For this review, take the finished solid that the model builds, in its own axes (mm). A direction names the side the tool comes from. Give positions to 0.01 mm unless a question says otherwise; leave off trailing zeros. Write each loop counter-clockwise with the first axis right and the second up, starting at its lowest first coordinate (ties: lowest second). Pieces come first, ordered by that corner, then holes.
Q1. Mouldability with a two-part tool opening along X and no side actions: class faces 3 (the cylindrical face through (-2.909, 0.042, -2.202)), 4 (the cylindrical face through (-5.58, 0.04, 0.02)), 5 (the flat face through (0, -3, 0)) as released by +X, released by -X, zero draft, split by the parting line, or undercut.
Q2. Insertion check: P1, Ø3, axis at x = -1, z = 0, coming from the -Y side; P2, Ø2, axis at x = -4.5, z = -2.5, coming from the -Y side; P3, Ø2, axis at x = -0.5, y = 9.5, coming from the -Z side; P4, Ø1, axis at x = -2.5, y = 0, coming from the +Z side. Each pin has a flat end and moves straight along its axis. Give the tip position at first contact, or say it passes through.
Q3. We need section C-C (y = 3.5). Write out the cut boundary in (x, z) (3 decimals).
Q4. Machinability: for faces 1 (the flat face through (-5, -3, 0)), 2 (the flat face through (-2, 3, 0)), which of the approach directions +Z, -Z, +X, -X, +Y, -Y give a long, thin tool a straight path to every point of the face, cutting with its end or side? Answer none if there is none.
Q5. For line 1 (Y direction, x = -1.5, z = -3.75); line 2 (Z direction, x = -6, y = 9); line 3 (Z direction, x = -1.25, y = 9.25), list the stretches that pass through material, from the lowest coordinate up.
Q6. We need section B-B (y = -1.5). Write out the cut boundary in (x, z).
Q7. We need section A-A (x = -2.54). Write out the cut boundary in (y, z) (3 decimals).
Q8. We need section D-D (z = -2.54). Write out the cut boundary in (x, y).
```python
from build123d import *

# Parameters (mm, degrees)
BOSS_EXTRUDE_1_DEPTH = 8.7
SKETCH_2_R           = 0.5
BOSS_EXTRUDE_2_DEPTH = 6


with BuildPart() as part:
    # Sketch 1 → Boss-Extrude 1 (new body)
    with BuildSketch(Plane.ZX.offset(3)):
        with BuildLine():
            Line((-0.13, 1.4), (2.03, 1.4))
            Line((2.03, 1.4), (2.03, -6.47))
            Line((2.03, -6.47), (-0.13, -6.47))
            ThreePointArc((-0.13, -6.47), (-4.065, -2.535), (-0.13, 1.4))
        make_face()
    extrude(amount=BOSS_EXTRUDE_1_DEPTH)

    # Sketch 2 → Boss-Extrude 2 (add)
    with BuildSketch(Plane.XZ.offset(-3)):
        Circle(SKETCH_2_R)
        with Locations((-2.54, -2.54)):
            Circle(SKETCH_2_R)
        with Locations((-5.08, 0)):
            Circle(SKETCH_2_R)
    extrude(amount=BOSS_EXTRUDE_2_DEPTH)


solid = part.part
```
Computed:
1. face 3: split by the parting line
1. face 4: undercut
1. face 5: zero draft
2. P1: stops at y = -3
2. P2: stops at y = 3
2. P3: stops at z = -3.93
2. P4: stops at z = -2.04
3. outline: (-6.47, -0.13) arc R3.935 ccw to (1.4, -0.13) - (1.4, 2.03) - (-6.47, 2.03) - close
4. face 1: +Z, -Z, +X, -X, -Y
4. face 2: -Y
5. line 1: y = 3 to 11.7
5. line 2: z = -1.99 to 2.03
5. line 3: z = -3.85 to 2.03
6. outline: circle Ø1 at (-5.08, 0); circle Ø1 at (-2.54, -2.54); circle Ø1 at (0, 0)
7. outline: (-3, -3.04) - (3, -3.04) - (3, -4.065) - (11.7, -4.065) - (11.7, 2.03) - (3, 2.03) - (3, -2.04) - (-3, -2.04) - close
8. outline: (-5.65, 3) - (-3.04, 3) - (-3.04, -3) - (-2.04, -3) - (-2.04, 3) - (0.58, 3) - (0.58, 11.7) - (-5.65, 11.7) - close
